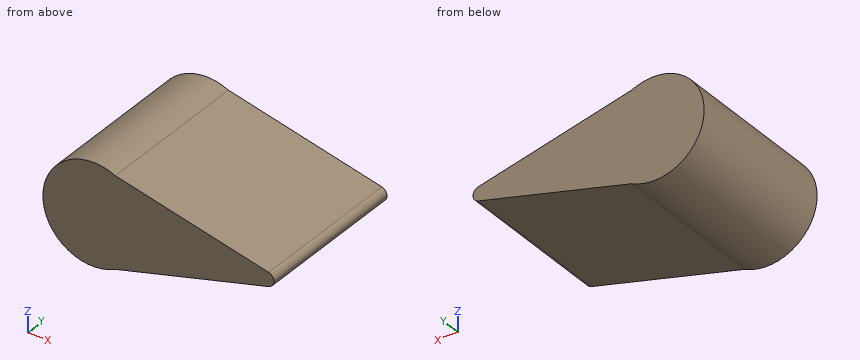
from build123d import *

# Parameters (mm, degrees)
F1_DEPTH = 57.32141


with BuildPart() as f1:
    # F0 (on Front) → F1 (new body)
    with BuildSketch(Plane.XZ):
        with BuildLine():
            ThreePointArc((7.854603, 16.062915), (15.168325, 9.467519), (17.880493, 0))
            ThreePointArc((17.880493, 0), (15.168325, -9.467519), (7.854603, -16.062915))
            Line((7.854603, -16.062915), (62.286771, -2.442561))
            ThreePointArc((62.286771, -2.442561), (59.15771, 0), (62.286771, 2.442561))
            Line((62.286771, 2.442561), (7.854603, 16.062915))
        make_face()
        with BuildLine():
            ThreePointArc((64.193446, 0), (63.660341, 1.549315), (62.286771, 2.442561))
            ThreePointArc((62.286771, 2.442561), (59.15771, 0), (62.286771, -2.442561))
            ThreePointArc((62.286771, -2.442561), (63.660341, -1.549315), (64.193446, 0))
        make_face()
        with BuildLine():
            ThreePointArc((7.854603, -16.062915), (15.168325, -9.467519), (17.880493, 0))
            ThreePointArc((17.880493, 0), (15.168325, 9.467519), (7.854603, 16.062915))
            ThreePointArc((7.854603, 16.062915), (-17.880493, 0), (7.854603, -16.062915))
        make_face()
    extrude(amount=F1_DEPTH)


solid = f1.part
Can you work these out from the model? Positions are in its coordinate system, mm. Coordinates: 2 decimals unless noted, no trailing zeros. Order: outer loops, then holes, each group sorted by start corner. A loop starts at its lowest first (then second) coordinate and runs counter-clockwise, first axis right, second up. Notation, with made-up numbers: (-9.75, 54.5) - (28.25, 54.5) arc R23 ccw to (28.25, 81.5) - close; hole circle Ø8 at (47.25, -14.75). An arc over 180 degrees is marked (long way). Answer as a JSON object with one key per item and string values. Group by question number.
Q1. Imagine slicing it at C-C (x = 48). Please give me the cut outline in (y, z).
Q2. Imagine slicing it at B-B (z = 12). Please give me the cut outline in (x, y).
Q3. Imagine slicing it at A-A (y = -42). Please give me the cut outline in (x, z).
Q4. I need wall thicknesses on line 1 (Z direction, x = 60, y = -28.5); line 2 (Z direction, x = 40, y = -51.5); line 3 (X direction, y = -6.5, z = 2). Which ranges of each line are inside material? Lowest first, please. Write a range as from..to.
Q5. Will these pins go through, and if not, where does the flat tip stop? P1, Ø3, axis at x = 40, y = -29.5, coming from the +Z side; P2, Ø6, axis at x = 27, y = -39, coming from the +Z side; P3, Ø10, axis at y = -7, z = -5.5, coming from the +X side.
Determined:
{
 "1": {"outline": "(-57.32, -6.02) - (0, -6.02) - (0, 6.02) - (-57.32, 6.02) - close"},
 "2": {"outline": "(-13.26, -57.32) - (24.09, -57.32) - (24.09, 0) - (-13.26, 0) - close"},
 "3": {"outline": "(7.85, -16.06) - (62.29, -2.44) arc R2.52 ccw to (64.19, 0) arc R2.52 ccw to (62.29, 2.44) - (7.85, 16.06) arc R17.88 ccw (long way) to start"},
 "4": {"line 1": "z = -3.01..3.01", "line 2": "z = -8.02..8.02", "line 3": "x = -17.77..63.21"},
 "5": {"P1": "stops at z = 8.39", "P2": "stops at z = 12.02", "P3": "stops at x = 64.14"}
}
